Geometry check sheet. Reference: drawing and pictorial views, mm from the part's lowest x, y, z. A direction names the side the tool comes from. Give positions to 0.01 mm unless a question says otherwise; leave off trailing zeros. Write each loop counter-clockwise with the first axis right and the second up, starting at its lowest first coordinate (ties: lowest second). Pieces come first, ordered by that corner, then holes. Notation, with made-up numbers: (57.25, -5.5) -> (62.25, -5.5) arc R16 cw to (62.25, 18.5) -> close; hole circle Ø7 at (23.5, 61). An arc over 180 degrees is marked (long way). Use a Markdown table: item, result. Add a question column.
1. Scan lines: probe 1 along Z at (x, y) = (14.5, 85); probe 2 along Z at (x, y) = (5, 84); probe 3 along X at (y, z) = (92.5, 19.5). Record each from-to range of solid material in increasing order. Write a range as [from, to].
2. Cross-section at C-C (y = 55.5). Enter the section's corners in (x, z), then the cut area to 3 significant figures.
3. Cross-section at D-D (z = 59). Enter the section's corners in (x, y), then the cut area to 3 significant figures.
4. Cross-section at B-B (x = 33). Enter the section's corners in (y, z), then the cut area to 3 significant figures.
5. Cross-section at A-A (z = 17.5). Enter the section's corners in (x, y).
6. Set-up check for the marked faces 1, 2 and 3: record each of +Z, -Z, +X, -X, +Y, -Y from which the full face is reachable in a straight line by a thin tool's end or side.
7. Gauge pin test, flat ends, axial feed: P1, Ø3, axis at x = 74, y = 72, coming from the +Z side; P2, Ø1, axis at x = 77.5, z = 32.5, coming from the -Y side; P3, Ø10, axis at y = 62.5, z = 43, coming from the -X side. Record the tip position at first contact, or that the pin passes through.
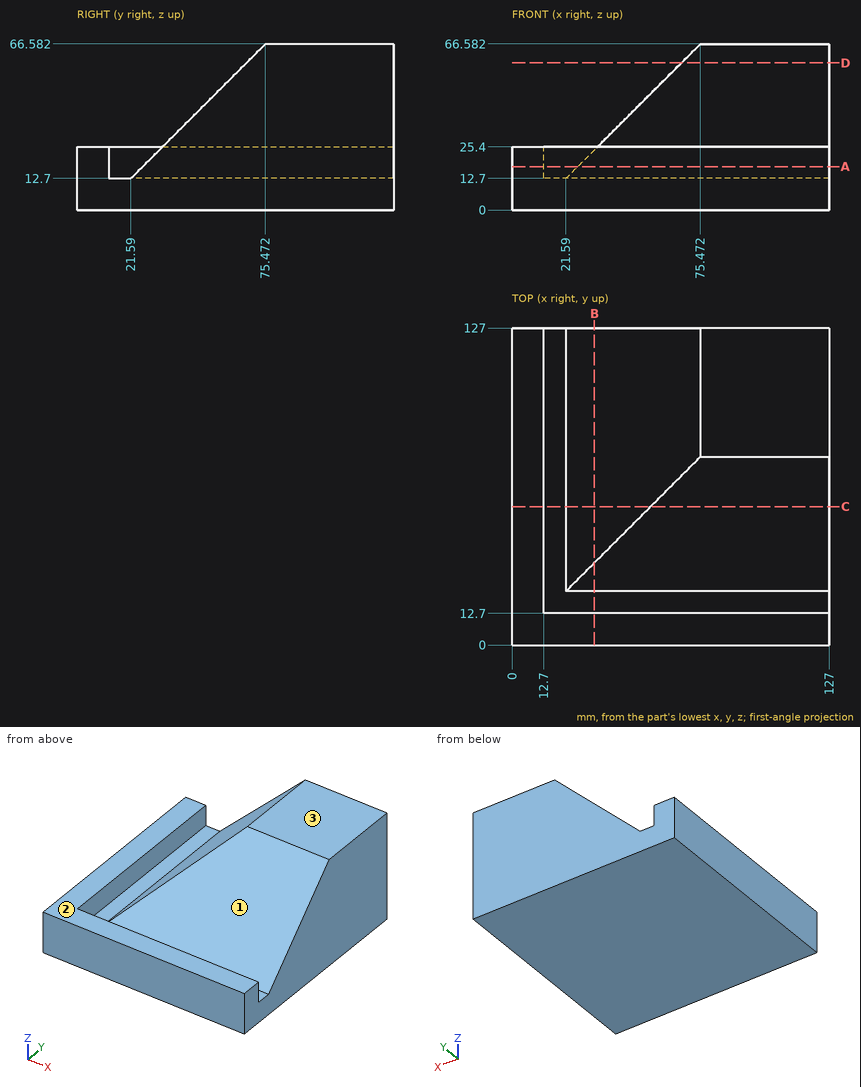
Worked answers:
| question | item | result |
|---|---|---|
| 1 | probe 1 | z = [0, 12.7] |
| 1 | probe 2 | z = [0, 25.4] |
| 1 | probe 3 | x = [0, 12.7], [28.39, 127] |
| 2 | outline | (0, 0) -> (127, 0) -> (127, 46.61) -> (55.5, 46.61) -> (21.59, 12.7) -> (12.7, 12.7) -> (12.7, 25.4) -> (0, 25.4) -> close |
| 2 | area | 4,770 mm² |
| 3 | outline | (67.89, 67.89) -> (127, 67.89) -> (127, 127) -> (67.89, 127) -> close |
| 3 | area | 3,490 mm² |
| 4 | outline | (0, 0) -> (127, 0) -> (127, 24.11) -> (33, 24.11) -> (21.59, 12.7) -> (12.7, 12.7) -> (12.7, 25.4) -> (0, 25.4) -> close |
| 4 | area | 2,910 mm² |
| 5 | outline | (0, 0) -> (127, 0) -> (127, 12.7) -> (12.7, 12.7) -> (12.7, 127) -> (0, 127) -> close; (26.39, 26.39) -> (127, 26.39) -> (127, 127) -> (26.39, 127) -> close |
| 6 | face 1 | +Z, +X |
| 6 | face 2 | +Z, -X, -Y |
| 6 | face 3 | +Z, +X, -X, +Y, -Y |
| 7 | P1 | stops at z = 64.61 |
| 7 | P2 | stops at y = 40.89 |
| 7 | P3 | stops at x = 46.89 |
